Source: CAD feature listing. Evaluate the final solid. Frame: model axes, mm. A direction names the side the tool comes from. Give positions to 0.01 mm unless a question says otherwise; leave off trailing zeros. Loops run counter-clockwise (first coordinate to the right, second up) from the corner with the lowest first, then second, coordinate; pieces in that order, holes last.
from build123d import *

# Parameters (mm, degrees)
SKETCH2_R           = 24.75
BOSS_EXTRUDE1_DEPTH = 4
SKETCH3_W           = 2.8
SKETCH3_H           = 2.45
BOSS_EXTRUDE2_DEPTH = 3.8
BOSS_EXTRUDE3_START = -6.3
SKETCH4_W           = 2.4
SKETCH4_H           = 2.45
BOSS_EXTRUDE3_DEPTH = 9.8


with BuildPart() as part:
    # Sketch2 → Boss-Extrude1 (new body)
    with BuildSketch(Plane.XY):
        with BuildLine():
            Line((-1.144859813, 35), (1.655140187, 35))
            Line((1.655140187, 35), (1.655140187, 26.19776729))
            ThreePointArc((1.655140187, 26.19776729), (-0.255503863, -26.2487565), (-1.144859813, 26.225022326))
            Line((-1.144859813, 26.225022326), (-1.144859813, 35))
        make_face()
        Circle(SKETCH2_R, mode=Mode.SUBTRACT)
    extrude(amount=BOSS_EXTRUDE1_DEPTH)

    # Sketch3 → Boss-Extrude2 (add)
    with BuildSketch(Plane(origin=(0, 0, 0), x_dir=(-1, 0, 0), z_dir=(0, 0, -1))):
        with Locations((-0.255140187, 33.775)):
            Rectangle(SKETCH3_W, SKETCH3_H)
    extrude(amount=BOSS_EXTRUDE2_DEPTH)

    # Sketch4 → Boss-Extrude3 (add)
    with BuildSketch(Plane(origin=(1.655140187, 0, 0), x_dir=(0, 0, -1), z_dir=(1, 0, 0)).offset(BOSS_EXTRUDE3_START)):
        with Locations((5, 33.775)):
            Rectangle(SKETCH4_W, SKETCH4_H)
    extrude(amount=BOSS_EXTRUDE3_DEPTH)


solid = part.part
1) Cut plane D-D (x = 20.5). Return loops of the section in (y, z), and give its area (3 significant figures).
Checks:
outline: (-16.4, 0) - (-13.87, 0) - (-13.87, 4) - (-16.4, 4) - close; (13.87, 0) - (16.4, 0) - (16.4, 4) - (13.87, 4) - close
area: 20.2 mm2
2) Cut plane B-B (x = 0). Return loops of the section in (y, z).
Checks:
outline: (-26.25, 0) - (-24.75, 0) - (-24.75, 4) - (-26.25, 4) - close; (24.75, 0) - (32.55, 0) - (32.55, -6.2) - (35, -6.2) - (35, 4) - (24.75, 4) - close
3) Cut plane A-A (y = 0). Return loops of the section in (x, z), and give its area (3 significant figures).
Checks:
outline: (-26.25, 0) - (-24.75, 0) - (-24.75, 4) - (-26.25, 4) - close; (24.75, 0) - (26.25, 0) - (26.25, 4) - (24.75, 4) - close
area: 12.0 mm2
4) Ray query, probe 1 along Y at (x, z) = (0, 1.2); probe 2 along X at (y, z) = (-10.5, 2.5); probe 3 along Y at (x, z) = (7, 3). Return the intervals inside material, ascending.
Checks:
probe 1: y = -26.25 to -24.75, 24.75 to 35
probe 2: x = -24.06 to -22.41, 22.41 to 24.06
probe 3: y = -25.3 to -23.74, 23.74 to 25.3
5) Cut plane C-C (z = 1). Return loops of the section in (x, y).
Checks:
outline: (-1.14, 26.23) arc R26.25 ccw (long way) to (1.66, 26.2) - (1.66, 35) - (-1.14, 35) - close; hole circle Ø49.5 at (0, 0)
6) Contact query for flat-ended pins moving along their axis: P1, Ø16, axis at x = 13, y = 17.5, coming from the -Z side; P2, Ø4, axis at y = 10, z = -1, coming from the -X side; P3, Ø2, axis at x = -2.5, y = 33.5, coming from the +Z side. Output: stop coordinate, or through.
Checks:
P1: stops at z = 0
P2: stops at x = -24.91
P3: stops at z = -3.8
7) Reachability of faces 4 (the flat face through (-1.145, 32, 1)), 5 (the flat face through (0, 32.55, -4)), 6 (the flat face through (3, 34, -3.8)) from +Z, -Z, +X, -X, +Y, -Y: full face, straight path, thin tool, end or side. Return the list, or none.
Checks:
face 4: +Z, -X, +Y
face 5: -Z, +X, -X, -Y
face 6: +Z, +X, +Y, -Y
8) Pull-direction query (X, two-part tool) for faces 1 (the flat face through (-3, 34, -3.8)), 2 (the cylindrical face through (-3.22, 24.54, 1.97)), 3 (the flat face through (1.655, 32, 1)); classes: released by +X, released by -X, zero draft, split by the parting line, or undercut.
Checks:
face 1: zero draft
face 2: undercut
face 3: released by +X
